Build history of the part. All positions in model axes, mm. A direction names the side the tool comes from. Give positions to 0.01 mm unless a question says otherwise; leave off trailing zeros. Order: outer loops, then holes, each group sorted by start corner. A loop starts at its lowest first (then second) coordinate and runs counter-clockwise, first axis right, second up. Notation, with made-up numbers: M 3.25,-12 L 24.25,-12 A7 ccw 24.25,-6 Z; hole C 27.5,-5 d1. An arc over 180 degrees is marked long. One line per item, written item: value. Start each with the question number.
from build123d import *

# Parameters (mm, degrees)
F0_R     = 3.048
F0_R_2   = 2.3749
F1_DEPTH = 5.4102
F2_START = 3.9624
F2_DEPTH = 21.4376


with BuildPart() as f1:
    # F0 (on Top) → F1 (new body)
    with BuildSketch(Plane.XY):
        with BuildLine():
            Line((28.9052, 6.5278), (0, 6.5278))
            ThreePointArc((0, 6.5278), (-5.1208699041, 4.048316226), (-6.351573493, -1.506548042))
            Line((-6.351573493, -1.506548042), (0.4261988754, -30.0814876494))
            ThreePointArc((0.4261988754, -30.0814876494), (4.2993416228, -32.7927187419), (7.4422, -29.2608))
            Line((7.4422, -29.2608), (7.4422, -8.0518))
            ThreePointArc((7.4422, -8.0518), (7.8885692655, -6.9741692655), (8.9662, -6.5278))
            Line((8.9662, -6.5278), (28.9052, -6.5278))
            ThreePointArc((28.9052, -6.5278), (29.4440153673, -6.3046153673), (29.6672, -5.7658))
            Line((29.6672, -5.7658), (29.6672, 5.7658))
            ThreePointArc((29.6672, 5.7658), (29.4440153673, 6.3046153673), (28.9052, 6.5278))
        make_face()
        Circle(F0_R, mode=Mode.SUBTRACT)
        with Locations((15.24, 0)):
            Circle(F0_R_2, mode=Mode.SUBTRACT)
        with Locations((15.24, 0)):
            Circle(F0_R_2)
    extrude(amount=F1_DEPTH)

    # F0 (on Top) → F2 (cut)
    with BuildSketch(Plane.XY.offset(F2_START)):
        with Locations((15.24, 0)):
            Circle(F0_R_2)
    extrude(amount=F2_DEPTH, mode=Mode.SUBTRACT)


solid = f1.part
1) Slice it at B-B (z = 2.5). List the corners of the cut face in (x, y).
2) Tool access for faces 4 (the cylindrical face through (14.931, 2.355, 4.676)), 5 (the flat face through (7.442, -19, 3)), 6 (the flat face through (29.667, 0, 3)): list every direction of +Z, -Z, +X, -X, +Y, -Y with a clear straight run to the whole face (end or side of a thin tool).
3) Slice it at D-D (y = -5). List the corners of the cut face in (x, z).
4) Pull direction Y, two halves, no side cores. Call faces 1 (the cylindrical face through (7.877, -6.986, 2.667)), 2 (the cylindrical face through (-0.4, 3.02, 2.67)), 3 (the cylindrical face through (-5.07, 4.11, 2.67)): pulls with the +Y half, pulls with the -Y half, needs draft (parallel to the pull), parting line crosses it, or undercut.
5) Slice it at C-C (x = 15.24). List the corners of the cut face in (y, z).
6) Slice it at A-A (y = 0). List the corners of the cut face in (x, z).
7) Drop flat-ended pins along their axis: P1, Ø2, axis at x = 17.5, z = 2.5, coming from the -Y side; P2, Ø1.4, axis at x = 14.5, y = -0.5, coming from the +Z side; P3, Ø1.6, axis at y = -22.5, z = 2.5, coming from the +X side. Give the stop position or say it passes through.
8) Drill centre lines: line 1 (Y direction, x = 15.24, z = 4.55); line 2 (Y direction, x = 9, z = 3.4); line 3 (Y direction, x = 2, z = 1.5). Where is each one in solid material? Low to high.
Results list:
1. outline: M -6.35,-1.51 L 0.43,-30.08 A3.56 ccw 7.44,-29.26 L 7.44,-8.05 A1.52 cw 8.97,-6.53 L 28.91,-6.53 A0.76 ccw 29.67,-5.77 L 29.67,5.77 A0.76 ccw 28.91,6.53 L 0,6.53 A6.53 ccw Z; hole C 0,0 d6.1
2. face 4: +Z
2. face 5: +Z, -Z, +X, -Y
2. face 6: +Z, -Z, +X, +Y, -Y
3. outline: M -5.52,0 L 29.67,0 L 29.67,5.41 L -5.52,5.41 Z
4. face 1: pulls with the -Y half
4. face 2: undercut
4. face 3: parting line crosses it
5. outline: M -6.53,0 L 6.53,0 L 6.53,5.41 L 2.37,5.41 L 2.37,3.96 L -2.37,3.96 L -2.37,5.41 L -6.53,5.41 Z
6. outline: M -6.53,0 L -3.05,0 L -3.05,5.41 L -6.53,5.41 Z; M 3.05,0 L 29.67,0 L 29.67,5.41 L 17.61,5.41 L 17.61,3.96 L 12.87,3.96 L 12.87,5.41 L 3.05,5.41 Z
7. P1: stops at y = -6.53
7. P2: stops at z = 3.96
7. P3: stops at x = 7.44
8. line 1: y = -6.53 to -2.37, 2.37 to 6.53
8. line 2: y = -6.53 to 6.53
8. line 3: y = -32.28 to -2.3, 2.3 to 6.53
